from build123d import *

# Parameters (mm, degrees)
SKETCH1_R           = 3.175
BOSS_EXTRUDE1_DEPTH = 17.272
CUT_EXTRUDE2_REACH  = 615.668
SKETCH3_R           = 3.175


with BuildPart() as part:
    # Sketch1 → Boss-Extrude1 (new body)
    with BuildSketch(Plane.XY):
        with BuildLine():
            Line((-563.971524104, 152.4), (563.971524104, 152.4))
            ThreePointArc((563.971524104, 152.4), (549.804304053, 197.496499323), (532.037545668, 241.3))
            Line((532.037545668, 241.3), (-532.037545668, 241.3))
            ThreePointArc((-532.037545668, 241.3), (-549.804304053, 197.496499323), (-563.971524104, 152.4))
        make_face()
        with Locations((533.201525575, 187.325)):
            Circle(SKETCH1_R, mode=Mode.SUBTRACT)
        with Locations((526.121546674, 206.375)):
            Circle(SKETCH1_R, mode=Mode.SUBTRACT)
        with Locations((-533.201525575, 187.325)):
            Circle(SKETCH1_R, mode=Mode.SUBTRACT)
        with Locations((-526.121546674, 206.375)):
            Circle(SKETCH1_R, mode=Mode.SUBTRACT)
    extrude(amount=BOSS_EXTRUDE1_DEPTH)

    # Sketch3 → Cut-Extrude2 (cut, up to next)
    with BuildSketch(Plane.XY.offset(17.272), mode=Mode.PRIVATE) as cut_extrude2_sk1:
        with Locations((152.4, 196.85)):
            Circle(SKETCH3_R)
    cut_extrude2_tool1 = extrude(cut_extrude2_sk1.sketch, amount=-CUT_EXTRUDE2_REACH, mode=Mode.PRIVATE) & part.part
    # Sketch3 → Cut-Extrude2 (cut, up to next)
    with BuildSketch(Plane.XY.offset(17.272), mode=Mode.PRIVATE) as cut_extrude2_sk2:
        with Locations((-152.4, 196.85)):
            Circle(SKETCH3_R)
    cut_extrude2_tool2 = extrude(cut_extrude2_sk2.sketch, amount=-CUT_EXTRUDE2_REACH, mode=Mode.PRIVATE) & part.part
    add(cut_extrude2_tool1.solids().sort_by_distance((152.4, 196.85, 17.272))[0], mode=Mode.SUBTRACT)
    add(cut_extrude2_tool2.solids().sort_by_distance((-152.4, 196.85, 17.272))[0], mode=Mode.SUBTRACT)


solid = part.part
Design review of the part built by this model. Coordinates are the model's own, in mm. Give positions to 0.01 mm unless a question says otherwise; leave off trailing zeros. Loops run counter-clockwise (first coordinate to the right, second up) from the corner with the lowest first, then second, coordinate; pieces in that order, holes last. Notation, with made-up numbers: (-25, 56.25) - (30, 56.25) arc R24 cw to (30, 91.25) - close; hole circle Ø11 at (-29, 86). An arc over 180 degrees is marked (long way). Use CSV: the item, a comma, the result in double quotes. Start each with the question number.
1. Add section A-A (z = 5.75). State the section outline as (x, y) points (3 decimals), plus the area to 3 significant figures.
2. Insertion check: P1, Ø4, axis at x = 526.12, y = 206.38, coming from the -Z side; P2, Ø1, axis at y = 231.5, z = 13.5, coming from the +X side; P3, Ø5, axis at y = 195, z = 3.5, coming from the +X side; P4, Ø1, axis at y = 184, z = 14, coming from the -X side. Each pin has a flat end and moves straight along its axis. Give the tip position at first contact, or say it passes through.
3. Wall thickness on L1, parallel to X at y = 188.5, z = 10.75; L2, parallel to X at y = 196.85, z = 8.5 (3 decimals); L3, parallel to X at y = 213.5, z = 3.75: over which ranges is each line inside the solid? List them lowest first.
Results found:
1,outline,"(-563.972, 152.4) - (563.972, 152.4) arc R584.2 ccw to (532.038, 241.3) - (-532.038, 241.3) arc R584.2 ccw to start; hole circle Ø6.35 at (-533.202, 187.325); hole circle Ø6.35 at (-526.122, 206.375); hole circle Ø6.35 at (-152.4, 196.85); hole circle Ø6.35 at (152.4, 196.85); hole circle Ø6.35 at (526.122, 206.375); hole circle Ø6.35 at (533.202, 187.325)"
1,area,"97,500 mm²"
2,P1,"passes through"
2,P2,"stops at x = 536.59"
2,P3,"stops at x = 551.57"
2,P4,"stops at x = -554.63"
3,L1,"x = -552.95 to -536.15, -530.25 to 530.25, 536.15 to 552.95"
3,L2,"x = -550.036 to -155.575, -149.225 to 149.225, 155.575 to 550.036"
3,L3,"x = -543.79 to 543.79"
